```python
from build123d import *

# Parameters (mm, degrees)
F1_DEPTH = 40
F3_DEPTH = 40
F4_W     = 10
F4_H     = 20
F5_DEPTH = 20
F7_DEPTH = 20
F9_DEPTH = 20


with BuildPart() as f1:
    # F0 (on Front) → F1 (new body)
    with BuildSketch(Plane.XZ):
        Polygon((0, 40), (0, 0), (50, 0), (50, 20), (30, 20), (30, 40), align=None)
    extrude(amount=F1_DEPTH)

    # F2 (on face) → F3 (cut)
    with BuildSketch(Plane.XY.offset(40)):
        with BuildLine():
            ThreePointArc((19.502008, -40), (0.089083, -19.972422), (19.55875, 0))
            Line((19.55875, 0), (0, 0))
            Line((0, 0), (0, -40))
            Line((0, -40), (19.502008, -40))
        make_face()
    extrude(amount=-F3_DEPTH, mode=Mode.SUBTRACT)

    # F4 (on face) → F5 (cut)
    with BuildSketch(Plane.XY.offset(40)):
        with Locations((25, -20)):
            Rectangle(F4_W, F4_H)
    extrude(amount=-F5_DEPTH, mode=Mode.SUBTRACT)

    # F6 (on face) → F7 (cut)
    with BuildSketch(Plane.XY.offset(40)):
        with BuildLine():
            Line((20, -30), (20, -10))
            ThreePointArc((20, -10), (10, -20), (20, -30))
        make_face()
    extrude(amount=-F7_DEPTH, mode=Mode.SUBTRACT)

    # F8 (on face) → F9 (cut)
    with BuildSketch(Plane.XY.offset(20)):
        with BuildLine():
            Line((50, -30), (50, -10))
            ThreePointArc((50, -10), (40, -20), (50, -30))
        make_face()
    extrude(amount=-F9_DEPTH, mode=Mode.SUBTRACT)


solid = f1.part
```
Source: CAD feature listing. Evaluate the final solid. Frame: model axes, mm. A direction names the side the tool comes from. Coordinates: 2 decimals unless noted, no trailing zeros. Write each loop counter-clockwise with the first axis right and the second up, starting at its lowest first coordinate (ties: lowest second). Pieces come first, ordered by that corner, then holes. Notation, with made-up numbers: (-25, 38) -> (7, 38) arc R24 ccw to (7, 52) -> close; hole circle Ø5 at (23.5, 35.25). An arc over 180 degrees is marked (long way). Return JSON: item names as keys, results as strings. Group by question number.
1) Section query D-D, the plane x = 47.5. Return loops of the section in (y, z).
2) Section query A-A, the plane x = 29. Return loops of the section in (y, z).
3) Contact query for flat-ended pins moving along their axis: P1, Ø1, axis at x = 14, y = -5.5, coming from the -Z side; P2, Ø8, axis at y = -3.5, z = 27.5, coming from the +X side; P3, Ø1, axis at y = -18, z = 10.5, coming from the +X side; P4, Ø6, axis at x = 14.5, z = 4.5, coming from the +Y side. Output: stop coordinate, or through.
4) Section query B-B, the plane z = 11.5. Return loops of the section in (x, y).
5) Set-up query: faces 5 (the face through (50, -35, 10)), 6 (the face through (25, -30, 30)), 7 (the face through (30, -5, 30)). Return all of +Z, -Z, +X, -X, +Y, -Y with unobstructed straight access to the full face (end or side cutting, diameter ignored); none if empty.
6) Ray query, line 1 along Z through (x, y) = (32, -11.5); line 2 along Y through (x, z) = (15, 37); line 3 along X through (y, z) = (-24.5, 8.5). Return the intervals inside material, ascending.
7) Section query C-C, the plane y = -20. Return loops of the section in (x, z).
8) Mould query, pull axis Y, two halves, no side actions, for faces 1 (the face through (0.093, -20.404, 20.28)), 2 (the face through (30, -20, 20)), 3 (the face through (31, -40, 16)), 4 (the face through (30, -35, 30)). Classes: +Y half, -Y half, draft (parallel to the pull), parting line (faces both ways), or undercut.
From the geometry:
{
 "1": {"outline": "(-40, 0) -> (-29.68, 0) -> (-29.68, 20) -> (-40, 20) -> close; (-10.32, 0) -> (0, 0) -> (0, 20) -> (-10.32, 20) -> close"},
 "2": {"outline": "(-40, 0) -> (0, 0) -> (0, 40) -> (-10, 40) -> (-10, 20) -> (-30, 20) -> (-30, 40) -> (-40, 40) -> close"},
 "3": {"P1": "z = 0", "P2": "x = 30", "P3": "x = 40.32", "P4": "y = -0.16"},
 "4": {"outline": "(19.5, -40) -> (50, -40) -> (50, -30) arc R10 cw to (50, -10) -> (50, 0) -> (19.56, 0) arc R20.01 ccw to start"},
 "5": {"face 5": "+Z, -Z, +X, +Y, -Y", "face 6": "+Z, +X", "face 7": "+Z, +X, +Y, -Y"},
 "6": {"line 1": "0 to 20", "line 2": "-39.35 to -28.66, -11.34 to -0.65", "line 3": "0.6 to 41.07"},
 "7": {"outline": "(0.09, 0) -> (40, 0) -> (40, 20) -> (10, 20) -> (10, 40) -> (0.09, 40) -> close"},
 "8": {"face 1": "parting line", "face 2": "undercut", "face 3": "-Y half", "face 4": "draft"}
}
